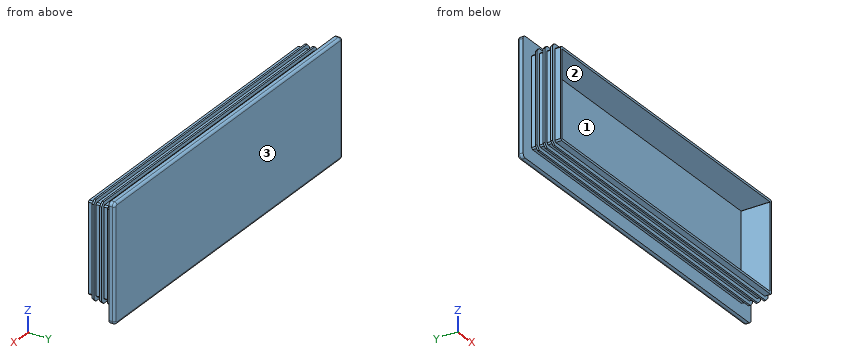
from build123d import *

# Parameters (mm, degrees)
SKETCH1_W           = 144.018
SKETCH1_H           = 42.418
BOSS_EXTRUDE1_DEPTH = 12.7
BOSS_EXTRUDE2_DEPTH = 2.54
CHAMFER1_SIZE       = 1.524
SHELL1_T            = -2.54
SKETCH4_W           = 1.524
SKETCH4_H           = 2.6035
FILLET2_R           = 1.016


with BuildPart() as part:
    # Sketch1 → Boss-Extrude1 (new body)
    with BuildSketch(Plane(origin=(0, 0, 0), x_dir=(1, 0, 0), z_dir=(0, 1, 0))):
        Rectangle(SKETCH1_W, SKETCH1_H)
    extrude(amount=BOSS_EXTRUDE1_DEPTH)

    # Sketch2 → Boss-Extrude2 (add)
    with BuildSketch(Plane(origin=(0, 12.7, 0), x_dir=(1, 0, 0), z_dir=(0, 1, 0))):
        with BuildLine():
            Line((-76.2, 23.876), (-76.2, -23.876))
            ThreePointArc((-76.2, -23.876), (-75.753630735, -24.953630735), (-74.676, -25.4))
            Line((-74.676, -25.4), (74.676, -25.4))
            ThreePointArc((74.676, -25.4), (75.753630735, -24.953630735), (76.2, -23.876))
            Line((76.2, -23.876), (76.2, 23.876))
            ThreePointArc((76.2, 23.876), (75.753630735, 24.953630735), (74.676, 25.4))
            Line((74.676, 25.4), (-74.676, 25.4))
            ThreePointArc((-74.676, 25.4), (-75.753630735, 24.953630735), (-76.2, 23.876))
        make_face()
    extrude(amount=BOSS_EXTRUDE2_DEPTH)

    # Chamfer1
    chamfer1_edges = [part.edges().sort_by_distance(p)[0] for p in [
        (72.009, 6.35, 21.209),
        (-72.009, 6.35, 21.209),
        (-72.009, 6.35, -21.209),
        (72.009, 6.35, -21.209),
    ]]
    chamfer(chamfer1_edges, length=CHAMFER1_SIZE)

    # Shell1
    shell1_openings = [part.faces().sort_by_distance(p)[0] for p in [
        (0, 0, 0),
    ]]
    offset(amount=SHELL1_T, openings=shell1_openings, kind=Kind.INTERSECTION)

    # Cut-Sweep2: sweep along a path in Sketch3
    with BuildLine(Plane(origin=(0, 0, 0), x_dir=(-1, 0, 0), z_dir=(0, -1, 0))) as cut_sweep2_path:
        Line((-72.009, 19.685), (-72.009, -19.685))
        Line((-72.009, -19.685), (-70.485, -21.209))
        Line((-70.485, -21.209), (70.485, -21.209))
        Line((70.485, -21.209), (72.009, -19.685))
        Line((72.009, -19.685), (72.009, 19.685))
        Line((72.009, 19.685), (70.485, 21.209))
        Line((70.485, 21.209), (-70.485, 21.209))
        Line((-70.485, 21.209), (-72.009, 19.685))
    # Sketch4 → Cut-Sweep2 (sweep, cut)
    with BuildSketch(Plane.XY):
        with Locations((71.247, 1.30175)):
            Rectangle(SKETCH4_W, SKETCH4_H)
        with Locations((71.247, 8.03275)):
            Rectangle(SKETCH4_W, SKETCH4_H)
        with Locations((71.247, 11.39825)):
            Rectangle(SKETCH4_W, SKETCH4_H)
        with Locations((71.247, 4.66725)):
            Rectangle(SKETCH4_W, SKETCH4_H)
    sweep(path=cut_sweep2_path.line, transition=Transition.RIGHT, mode=Mode.SUBTRACT)

    # Fillet2
    fillet2_edges = [part.edges().sort_by_distance(p)[0] for p in [
        (-75.753630735, 15.24, 24.953630735),
        (0, 15.24, 25.4),
        (75.753630735, 15.24, 24.953630735),
        (76.2, 15.24, 0),
        (75.753630735, 15.24, -24.953630735),
        (0, 15.24, -25.4),
        (-75.753630735, 15.24, -24.953630735),
        (-76.2, 15.24, 0),
    ]]
    fillet(fillet2_edges, radius=FILLET2_R)


solid = part.part
Part model, mm, in its own coordinate system. Face numbers are marked on the shaded views. Coordinates: 2 decimals unless noted, no trailing zeros. Use a Markdown table: item, result. Add a question column.
Item 1: Probe probe 1 along Y at (x, z) = (17, -20); probe 2 along Z at (x, y) = (68, 9) (3 decimals); probe 3 along X at (y, z) = (10.75, -3.5) (3 decimals). List the from-to ranges inside material, lowest first.
Item 2: Pull direction X, two halves, no side cores. Call the marked faces 1, 2 and 3: +X half, -X half, draft (parallel to the pull), parting line (faces both ways), or undercut.
Item 3: Flat gauge pins, fed straight in: P1, Ø3, axis at y = 9.5, z = 5, coming from the -X side; P2, Ø1.5, axis at x = -17.5, y = 3, coming from the +Z side; P3, Ø0.8, axis at x = 1.5, y = 3, coming from the -Z side. Where does each tip first touch, or does it go through?
Geometry says:
| question | item | result |
|---|---|---|
| 1 | probe 1 | 2.6 to 3.37, 5.97 to 6.73, 9.33 to 10.1, 12.7 to 15.24 |
| 1 | probe 2 | -19.685 to -18.669, 18.669 to 19.685 |
| 1 | probe 3 | -70.485 to -69.469, 69.469 to 70.485 |
| 2 | face 1 | undercut |
| 2 | face 2 | undercut |
| 2 | face 3 | draft |
| 3 | P1 | x = -72.01 |
| 3 | P2 | z = 21.21 |
| 3 | P3 | z = -21.21 |
